The model under review builds one solid part; all positions refer to its coordinate system, in mm. Coordinates: 2 decimals unless noted, no trailing zeros. Order: outer loops, then holes, each group sorted by start corner. A loop starts at its lowest first (then second) coordinate and runs counter-clockwise, first axis right, second up. Notation, with made-up numbers: M -32.5,-4.75 L 18.5,-4.75 A26 cw 18.5,11.25 Z; hole C -11.75,45 d11. An arc over 180 degrees is marked long. Write each question's results on one line, items separated by ' | '.
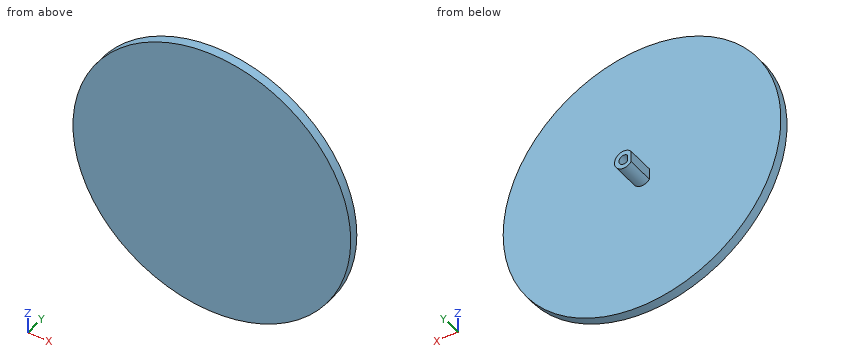
from build123d import *

# Parameters (mm, degrees)
SKETCH1_R           = 75
BOSS_EXTRUDE1_DEPTH = 5
BOSS_EXTRUDE2_DEPTH = 15


with BuildPart() as part:
    # Sketch1 → Boss-Extrude1 (new body)
    with BuildSketch(Plane(origin=(0, 0, 0), x_dir=(1, 0, 0), z_dir=(0, 1, 0))):
        Circle(SKETCH1_R)
    extrude(amount=BOSS_EXTRUDE1_DEPTH)

    # Sketch3 → Boss-Extrude2 (add)
    with BuildSketch(Plane(origin=(0, 5, 0), x_dir=(1, 0, 0), z_dir=(0, 1, 0))):
        with BuildLine():
            Line((-4, 3), (-4, -3))
            ThreePointArc((-4, -3), (5, 0), (-4, 3))
        make_face()
        with BuildLine():
            Line((-2.1, 1.532970972), (-2.1, -1.532970972))
            ThreePointArc((-2.1, -1.532970972), (2.6, 0), (-2.1, 1.532970972))
        make_face(mode=Mode.SUBTRACT)
    extrude(amount=BOSS_EXTRUDE2_DEPTH)


solid = part.part
1) Take a section at A-A on x = 0. State the section outline as (y, z) points.
Solutions:
outline: M 0,-75 L 5,-75 L 5,-5 L 20,-5 L 20,-2.6 L 5,-2.6 L 5,2.6 L 20,2.6 L 20,5 L 5,5 L 5,75 L 0,75 Z
2) Take a section at D-D on z = -23.5. State the section outline as (x, y) points, plus the area to 3 significant figures.
Solutions:
outline: M -71.22,0 L 71.22,0 L 71.22,5 L -71.22,5 Z | area: 712 mm2
3) Take a section at B-B on y = 7.5. State the section outline as (x, z) points, plus the area to 3 significant figures.
Solutions:
outline: M -4,-3 A5 ccw long -4,3 Z; hole M -2.1,-1.53 A2.6 ccw long -2.1,1.53 Z | area: 54.3 mm2
4) For pin 1 (8 mm diameter, centred on x = -40, y = 3, fed in from -Z); pin 2 (5 mm diameter, centred on y = 10.5, z = 0, fed in from -X); pin 3 (4 mm diameter, centred on x = 18, z = 58, fed in from +Y), all flat-tipped, find the tip position at first contact; note any pin that passes through.
Solutions:
pin 1: z = -65.8 | pin 2: x = -4 | pin 3: y = 5
5) To check wall thickness, follow line 1 along Z through (x, y) = (0, 12); line 2 along Y through (x, z) = (-59, 32); line 3 along Z through (x, y) = (8.5, 2.25). State the ranges of each line that lie inside material, in increasing order.
Solutions:
line 1: -5 to -2.6, 2.6 to 5 | line 2: 0 to 5 | line 3: -74.52 to 74.52
6) Take a section at C-C on z = -58. State the section outline as (x, y) points.
Solutions:
outline: M -47.55,0 L 47.55,0 L 47.55,5 L -47.55,5 Z
